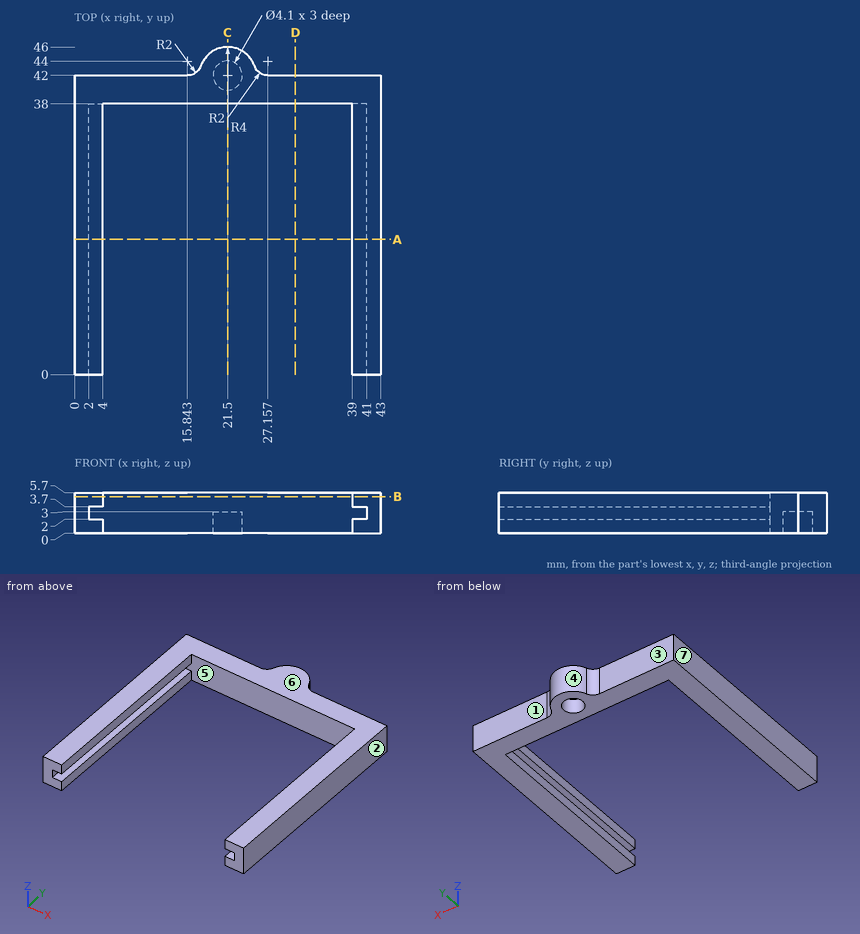
Check sheet for the drawn part. Datum: minimum x, y, z corner. Units: mm. A direction names the side the tool comes from. Round coordinates to 2 decimals unless told otherwise and drop trailing zeros. Order: outer loops, then holes, each group sorted by start corner. A loop starts at its lowest first (then second) coordinate and runs counter-clockwise, first axis right, second up.
1. Go/stop test with flat-tipped pins: P1, Ø1.5, axis at x = 9, z = 1.5, coming from the -Y side; P2, Ø3, axis at x = 8.5, z = 2.5, coming from the +Y side. Record where each tip stops, or that it passes through.
Final values:
P1: stops at y = 38
P2: stops at y = 42
2. Access from +Z, -Z, +X, -X, +Y, -Y to the whole of each face (thin tool, end or side, straight path). Record for the marked faces 1, 2 and 3.
Final values:
face 1: +Z, -Z, +X, +Y
face 2: +Z, -Z, +X, +Y, -Y
face 3: +Z, -Z, -X, +Y
3. Section check A-A on y = 19. Record the cut outline in (x, z).
Final values:
outline: (0, 0) - (4, 0) - (4, 2) - (2, 2) - (2, 3.7) - (4, 3.7) - (4, 5.7) - (0, 5.7) - close; (39, 0) - (43, 0) - (43, 5.7) - (39, 5.7) - (39, 3.7) - (41, 3.7) - (41, 2) - (39, 2) - close
4. Thickness scan on L1, parallel to Y at x = 21.5, z = 0.8; L2, parallel to X at y = 32.5, z = 3.9; L3, parallel to Z at x = 40.5, y = 29. Record the ranges inside material, lowest first.
Final values:
L1: y = 38 to 39.95, 44.05 to 46
L2: x = 0 to 4, 39 to 43
L3: z = 0 to 2, 3.7 to 5.7
5. Section check B-B on z = 5.15. Record the cut outline in (x, y).
Final values:
outline: (0, 0) - (4, 0) - (4, 38) - (39, 38) - (39, 0) - (43, 0) - (43, 42) - (27.16, 42) arc R2 cw to (25.27, 43.33) arc R4 ccw to (17.73, 43.33) arc R2 cw to (15.84, 42) - (0, 42) - close
6. Release check for a two-part mould opening along X. For the marked faces 4, 5, 6 and 7 record: +X half, -X half, draft (parallel to the pull), parting line (faces both ways), or undercut.
Final values:
face 4: parting line
face 5: undercut
face 6: draft
face 7: -X half
7. Section check D-D on x = 31. Record the cut outline in (y, z).
Final values:
outline: (38, 0) - (42, 0) - (42, 5.7) - (38, 5.7) - close
8. Section check C-C on x = 21.5. Record the cut outline in (y, z), then the cut area to 3 significant figures.
Final values:
outline: (38, 0) - (39.95, 0) - (39.95, 3) - (44.05, 3) - (44.05, 0) - (46, 0) - (46, 5.7) - (38, 5.7) - close
area: 33.3 mm2
